Geometry check sheet. Reference: the model listing, model coordinates, mm. A direction names the side the tool comes from. Coordinates: 2 decimals unless noted, no trailing zeros. Loops run counter-clockwise (first coordinate to the right, second up) from the corner with the lowest first, then second, coordinate; pieces in that order, holes last. Notation, with made-up numbers: M -15,-20.5 L 18,-20.5 A28 ccw 18,1.5 Z; hole C 33,87.25 d2. An arc over 180 degrees is marked long. One line per question, with ' | ' between items. Start each with the question number.
from build123d import *

# Parameters (mm, degrees)
SKETCH148_W             = 15
SKETCH148_H             = 5.5
PAD032_DEPTH            = 6.75
BODY059_PLACEMENT_ANGLE = 180


with BuildPart() as part:
    # Sketch148 → Pad032 (new body, symmetric)
    with BuildSketch(Plane.XY):
        with Locations((0, -4.25)):
            Rectangle(SKETCH148_W, SKETCH148_H)
    extrude(amount=PAD032_DEPTH, both=True)

    # Sketch149 → Groove006 (revolve, cut)
    with BuildSketch(Plane.XY):
        Polygon((0, 0), (0, -8), (4, -8), (4, -4), (2, -4), (2, 0), align=None)
    revolve(axis=Axis((0, 0, 0), (0, 1, 0)), mode=Mode.SUBTRACT)

    # SubtractivePipe006003: sweep along a path in Sketch150
    with BuildLine(Plane.XZ) as subtractivepipe006003_path:
        ThreePointArc((6.75, 3), (0, 9.75), (-6.75, 3))
        Line((-6.75, 3), (-6.75, -3))
        ThreePointArc((-6.75, -3), (0, -9.75), (6.75, -3))
        Line((6.75, -3), (6.75, 3))
    # Sketch151 → SubtractivePipe006003 (sweep, cut)
    with BuildSketch(Plane.XY):
        Polygon((4.25, 0), (4.25, -3), (6.7, -3), (6.7, -8), (10, -8), (10, 0), align=None)
    sweep(path=subtractivepipe006003_path.line, mode=Mode.SUBTRACT)


with BuildPart() as part_1:
    # Body059 placement: moved
    add(part.part.moved(Location((50, 0, -1))).rotate(Axis((50, 0, -1), (0, 1, 0)), BODY059_PLACEMENT_ANGLE))


solid = part_1.part
1. Tool access check on faces 1 (the cylindrical face through (46.34, -2.26, -6.16)), 2 (the cylindrical face through (53.66, -2.26, 4.16)), 3 (the flat face through (54.25, -2, -1)). Record the directions out of +Z, -Z, +X, -X, +Y, -Y that give a thin tool (end or side, any length) a straight path to the whole face; none if there is none.
2. Thickness scan on line 1 (Z direction, x = 50, y = -2.7); line 2 (Z direction, x = 50, y = -6.4); line 3 (X direction, y = -4.9, z = -2.25). Record the ranges inside material, lowest first.
3. Sectioned sample at D-D (x = 54.75). Record the cut outline in (y, z).
4. Sectioned sample at C-C (z = -1). Record the cut outline in (x, y).
5. Sectioned sample at A-A (x = 50). Record the cut outline in (y, z).
6. Depth check by flat-ended pin: pin 1 Ø2.5 at (x, z) = (45, -3) entering from +Y; pin 2 Ø6.5 at (x, z) = (50, -1.5) entering from -Y; pin 3 Ø1.6 at (y, z) = (-2, -0.5) entering from +X; pin 4 Ø1.6 at (y, z) = (-2, -0.5) entering from -X. Enter the tip coordinate at first touch or a pass-through.
7. Sectioned sample at B-B (y = -5.65). Record the cut outline in (x, z).
8. Draft check along Z on faces 4 (the flat face through (50, -5, 5.75)), 5 (the flat face through (52, -4, -2)), 6 (the flat face through (55, -3, -1)), 7 (the cylindrical face through (53.63, -2.26, -6.21)). Enter one of: +Z half, -Z half, draft (parallel to the pull), parting line (faces both ways), or undercut.
Result:
1) face 1: -Z, -X, +Y | face 2: +Z, +X, +Y | face 3: +Z, -Z, +X, +Y
2) line 1: z = -7.75 to -3, 1 to 5.75 | line 2: z = -7.75 to -5, 3 to 5.75 | line 3: x = 43.3 to 46.2, 53.8 to 56.7
3) outline: M -7,-7.75 L -3,-7.75 L -3,5.75 L -7,5.75 Z
4) outline: M 43.3,-7 L 46,-7 L 46,-4 L 48,-4 L 48,-1.5 L 45.75,-1.5 L 45.75,-3 L 43.3,-3 Z; M 52,-4 L 54,-4 L 54,-7 L 56.7,-7 L 56.7,-3 L 54.25,-3 L 54.25,-1.5 L 52,-1.5 Z
5) outline: M -7,-7.75 L -1.5,-7.75 L -1.5,-3 L -4,-3 L -4,-5 L -7,-5 Z; M -7,3 L -4,3 L -4,1 L -1.5,1 L -1.5,5.75 L -7,5.75 Z
6) pin 1: stops at y = -1.5 | pin 2: stops at y = -4 | pin 3: stops at x = 54.25 | pin 4: stops at x = 45.75
7) outline: M 43.3,-4 A6.7 ccw 44.45,-7.75 L 55.55,-7.75 A6.7 ccw 56.7,-4 L 56.7,2 A6.7 ccw 55.55,5.75 L 44.45,5.75 A6.7 ccw 43.3,2 Z; hole C 50,-1 d8
8) face 4: +Z half | face 5: undercut | face 6: draft | face 7: -Z half
